from build123d import *

# Parameters (mm, degrees)
SKETCH1_R           = 15
BOSS_EXTRUDE1_DEPTH = 0.25
BOSS_EXTRUDE2_START = -20.32
SKETCH2_R           = 15
SKETCH2_R_2         = 12.815737343
BOSS_EXTRUDE2_DEPTH = 20.32
SKETCH3_R           = 4.490128061
BOSS_EXTRUDE3_DEPTH = 19.05
FILLET2_R           = 1.016


with BuildPart() as part:
    # Sketch1 → Boss-Extrude1 (new body)
    with BuildSketch(Plane(origin=(0, 0, 0), x_dir=(1, 0, 0), z_dir=(0, 1, 0))):
        with Locations(Location((0, 0, 0), (0, 0, 270))):
            Circle(SKETCH1_R)
        with BuildLine():
            Line((-12.801684406, 0.6), (-10.235182592, 0.6))
            ThreePointArc((-10.235182592, 0.6), (0, 10.252753907), (10.235182592, 0.6))
            Line((10.235182592, 0.6), (12.801684406, 0.6))
            ThreePointArc((12.801684406, 0.6), (0, 12.815737343), (-12.801684406, 0.6))
        make_face(mode=Mode.SUBTRACT)
        with BuildLine():
            Line((-0.6, 7.600213812), (-0.6, 5.084960781))
            ThreePointArc((-0.6, 5.084960781), (-5.120236922, 0), (-0.6, -5.084960781))
            Line((-0.6, -5.084960781), (-0.6, -7.600213812))
            ThreePointArc((-0.6, -7.600213812), (-7.623860569, 0), (-0.6, 7.600213812))
        make_face(mode=Mode.SUBTRACT)
        with BuildLine():
            Line((0.6, 5.084960781), (0.6, 7.600213812))
            ThreePointArc((0.6, 7.600213812), (7.623860569, 0), (0.6, -7.600213812))
            Line((0.6, -7.600213812), (0.6, -5.084960781))
            ThreePointArc((0.6, -5.084960781), (5.120236922, 0), (0.6, 5.084960781))
        make_face(mode=Mode.SUBTRACT)
        with BuildLine():
            Line((-12.801684406, -0.6), (-10.235182592, -0.6))
            ThreePointArc((-10.235182592, -0.6), (0, -10.252753907), (10.235182592, -0.6))
            Line((10.235182592, -0.6), (12.801684406, -0.6))
            ThreePointArc((12.801684406, -0.6), (0, -12.815737343), (-12.801684406, -0.6))
        make_face(mode=Mode.SUBTRACT)
    extrude(amount=BOSS_EXTRUDE1_DEPTH)

    # Sketch2 → Boss-Extrude2 (add)
    with BuildSketch(Plane(origin=(0, 0.25, 0), x_dir=(1, 0, 0), z_dir=(0, 1, 0)).offset(BOSS_EXTRUDE2_START)):
        with Locations(Location((0, 0, 0), (0, 0, 270))):
            Circle(SKETCH2_R)
        with Locations(Location((0, 0, 0), (0, 0, 2.683422553))):
            Circle(SKETCH2_R_2, mode=Mode.SUBTRACT)
    extrude(amount=BOSS_EXTRUDE2_DEPTH)

    # Sketch3 → Boss-Extrude3 (add)
    with BuildSketch(Plane.XZ):
        with Locations(Location((0, 0, 0), (0, 0, 90))):
            Circle(SKETCH3_R)
        Polygon((-1.524, 1.524), (-1.524, 2.667), (1.524, 2.667), (1.524, 1.524), (2.667, 1.524), (2.667, -1.524), (1.524, -1.524), (1.524, -2.667), (-1.524, -2.667), (-1.524, -1.524), (-2.667, -1.524), (-2.667, 1.524), align=None, mode=Mode.SUBTRACT)
    extrude(amount=BOSS_EXTRUDE3_DEPTH)

    # Fillet2
    # the kernel refuses this fillet: 1.016 mm, written as the material it adds along each edge
    with BuildSketch(Plane(origin=(0, 0, 0), x_dir=(0, 0, 1), z_dir=(1, 0, 0))) as fillet2_piece_1_section:
        with BuildLine():
            CenterArc((4.490128061 + FILLET2_R, FILLET2_R), FILLET2_R, 180, 90)
            Line((4.490128061, FILLET2_R), (4.490128061, 0))
            Line((4.490128061, 0), (4.490128061 + FILLET2_R, 0))
        make_face()
    fillet2_piece_1 = revolve(axis=Axis((0, 0, 0), (0, -1, 0)), mode=Mode.PRIVATE)
    fillet2_piece_1 = split(fillet2_piece_1, bisect_by=Plane(origin=(0.6, -0.022686873, 5.204418355), z_dir=(-1, 0, 0)), keep=Keep.TOP, mode=Mode.PRIVATE)
    fillet2_piece_1 = split(fillet2_piece_1, bisect_by=Plane(origin=(-0.6, -0.022686873, 5.204418355), z_dir=(1, 0, 0)), keep=Keep.TOP, mode=Mode.PRIVATE)
    add(fillet2_piece_1)
    with BuildSketch(Plane(origin=(0, 0, 0), x_dir=(0, 0, 1), z_dir=(1, 0, 0))) as fillet2_piece_2_section:
        with BuildLine():
            CenterArc((4.490128061 + FILLET2_R, FILLET2_R), FILLET2_R, 180, 90)
            Line((4.490128061, FILLET2_R), (4.490128061, 0))
            Line((4.490128061, 0), (4.490128061 + FILLET2_R, 0))
        make_face()
    fillet2_piece_2 = revolve(axis=Axis((0, 0, 0), (0, -1, 0)), mode=Mode.PRIVATE)
    fillet2_piece_2 = fillet2_piece_2 & Plane(origin=(0, -0.038068082, 0), x_dir=(0.11718207753036296, 0, 0.9931104473852181), z_dir=(0, -1, 0)) * Cylinder(5.120236922, 23, mode=Mode.PRIVATE)
    add(fillet2_piece_2)


solid = part.part
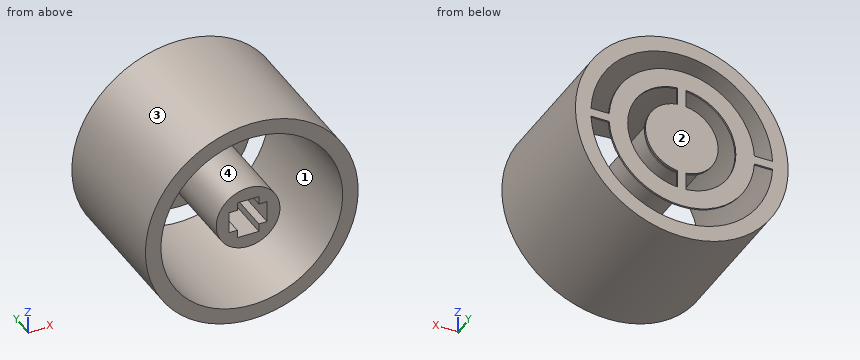
Check sheet for the modelled part. Datum: model origin and axes. Units: mm. Face numbers are marked on the shaded views. Give positions to 0.01 mm unless a question says otherwise; leave off trailing zeros. Write each loop counter-clockwise with the first axis right and the second up, starting at its lowest first coordinate (ties: lowest second). Pieces come first, ordered by that corner, then holes. Notation, with made-up numbers: (21, -6) -> (55, -6) arc R24 ccw to (55, 29) -> close; hole circle Ø7 at (48.5, 86.5). An arc over 180 degrees is marked (long way). Write item = value, one per line.
Item 1: Release check for a two-part mould opening along Z. For the marked faces 1, 2, 3 and 4 record: +Z half, -Z half, draft (parallel to the pull), parting line (faces both ways), or undercut.
Output:
face_1 = undercut
face_2 = draft
face_3 = parting line
face_4 = undercut
Item 2: Scan lines: probe 1 along X at (y, z) = (-7, 0); probe 2 along X at (y, z) = (-13.5, 3); probe 3 along Z at (x, y) = (-2.5, -12.25). Record each from-to range of solid material in increasing order. Write a range as from..to.
Output:
probe_1 = -15..-12.82, -4.49..-2.67, 2.67..4.49, 12.82..15
probe_2 = -14.7..-12.46, -3.34..3.34, 12.46..14.7
probe_3 = -14.79..-12.57, -3.73..-1.52, 1.52..3.73, 12.57..14.79
Item 3: Sectioned sample at A-A on y = -3.5. Record the boundary of the cut face in (x, z), and give its area (3 significant figures).
Output:
outline = circle Ø30 at (0, 0); circle Ø8.98 at (0, 0); hole circle Ø25.63 at (0, 0); hole (-2.67, -1.52) -> (-1.52, -1.52) -> (-1.52, -2.67) -> (1.52, -2.67) -> (1.52, -1.52) -> (2.67, -1.52) -> (2.67, 1.52) -> (1.52, 1.52) -> (1.52, 2.67) -> (-1.52, 2.67) -> (-1.52, 1.52) -> (-2.67, 1.52) -> close
area = 231 mm^2
Item 4: Gauge pin test, flat ends, axial feed: pin 1 (1 mm diameter, centred on x = -9.5, y = -12, fed in from -Z); pin 2 (2.5 mm diameter, centred on y = -12, z = -0.5, fed in from -X); pin 3 (0.9 mm diameter, centred on y = -11, z = -2, fed in from +X); pin 4 (5 mm diameter, centred on x = -7, y = -3, fed in from +Z). Record the tip position at first contact, or that the pin passes through.
Output:
pin_1 = -12
pin_2 = -15
pin_3 = 14.92
pin_4 = 14.31
Item 5: Sectioned sample at D-D on x = -6.5. Record the boundary of the cut face in (y, z), and give its area (3 significant figures).
Output:
outline = (-20.07, -13.52) -> (0.25, -13.52) -> (0.25, -11.05) -> (-20.07, -11.05) -> close; (-20.07, 11.05) -> (0.25, 11.05) -> (0.25, 13.52) -> (-20.07, 13.52) -> close; (0, -7.93) -> (0.25, -7.93) -> (0.25, -3.98) -> (0, -3.98) -> close; (0, 3.98) -> (0.25, 3.98) -> (0.25, 7.93) -> (0, 7.93) -> close
area = 102 mm^2
Item 6: Sectioned sample at B-B on z = 0. Record the boundary of the cut face in (x, y), and give its area (3 significant figures).
Output:
outline = (-15, -20.07) -> (-12.82, -20.07) -> (-12.82, 0) -> (-7.62, 0) -> (-7.62, 0.25) -> (-15, 0.25) -> close; (-5.12, -0.08) arc R1.02 cw to (-4.49, -1.02) -> (-4.49, -19.05) -> (-2.67, -19.05) -> (-2.67, 0) -> (2.67, 0) -> (2.67, -19.05) -> (4.49, -19.05) -> (4.49, -1.02) arc R1.02 cw to (5.12, -0.08) -> (5.12, 0.25) -> (-5.12, 0.25) -> close; (7.62, 0) -> (12.82, 0) -> (12.82, -20.07) -> (15, -20.07) -> (15, 0.25) -> (7.62, 0.25) -> close
area = 164 mm^2
Item 7: Sectioned sample at C-C on x = 12. Record the boundary of the cut face in (y, z), and give its area (3 significant figures).
Output:
outline = (-20.07, -9) -> (0.25, -9) -> (0.25, -4.5) -> (-20.07, -4.5) -> close; (-20.07, 4.5) -> (0.25, 4.5) -> (0.25, 9) -> (-20.07, 9) -> close; (0, -0.6) -> (0.25, -0.6) -> (0.25, 0.6) -> (0, 0.6) -> close
area = 183 mm^2
